Geometry: final body of the model. Coordinates: model frame, mm. A direction names the side the tool comes from. Give positions to 0.01 mm unless a question says otherwise; leave off trailing zeros. Order: outer loops, then holes, each group sorted by start corner. A loop starts at its lowest first (then second) coordinate and runs counter-clockwise, first axis right, second up. Notation, with made-up numbers: (63.25, 32.5) -> (103.25, 32.5) arc R18 cw to (103.25, 60.5) -> close; hole circle Ø10 at (48.5, 6). An arc over 180 degrees is marked (long way). Write item = value, one per line.
```python
from build123d import *

# Parameters (mm, degrees)
F0_W      = 96.012
F0_H      = 50.8
F1_DEPTH  = 56.896
F3_DEPTH  = 96.012
F5_DEPTH  = 56.896
F7_DEPTH  = 56.896
F9_DEPTH  = 31.75
F10_W     = 25.4
F10_H     = 25.4
F11_DEPTH = 19.304
F12_W     = 28.956
F12_H     = 20.32
F13_DEPTH = 13.716


with BuildPart() as f1:
    # F0 (on Front) → F1 (new body)
    with BuildSketch(Plane.XZ):
        with Locations((48.006, 25.4)):
            Rectangle(F0_W, F0_H)
    extrude(amount=F1_DEPTH)

    # F2 (on face) → F3 (cut)
    with BuildSketch(Plane.YZ.offset(96.012)):
        Polygon((-56.896, 6.604), (-12.7, 50.8), (-56.896, 50.8), align=None)
    extrude(amount=-F3_DEPTH, mode=Mode.SUBTRACT)

    # F4 (on face) → F5 (cut)
    with BuildSketch(Plane(origin=(0, 0, 0), x_dir=(-1, 0, 0), z_dir=(0, 1, 0))):
        Polygon((0, 32.004), (0, 50.8), (-57.955627, 50.8), (-25.4, 32.004), align=None)
    extrude(amount=-F5_DEPTH, mode=Mode.SUBTRACT)

    # F6 (on face) → F7 (cut)
    with BuildSketch(Plane(origin=(0, 0, 0), x_dir=(-1, 0, 0), z_dir=(0, 1, 0))):
        Polygon((-77.216, 50.8), (-96.012, 50.8), (-96.012, 32.004), align=None)
    extrude(amount=-F7_DEPTH, mode=Mode.SUBTRACT)

    # F8 (on face) → F9 (cut)
    with BuildSketch(Plane.YZ.offset(96.012)):
        with BuildLine():
            ThreePointArc((-19.304, 7.8105), (-13.69134, 10.13534), (-11.3665, 15.748))
            ThreePointArc((-11.3665, 15.748), (-24.91666, 21.36066), (-19.304, 7.8105))
        make_face()
    extrude(amount=-F9_DEPTH, mode=Mode.SUBTRACT)

    # F10 (on face) → F11 (cut)
    with BuildSketch(Plane.XZ.offset(56.896)):
        with Locations((83.312, 12.7)):
            Rectangle(F10_W, F10_H)
    extrude(amount=-F11_DEPTH, mode=Mode.SUBTRACT)

    # F12 (on face) → F13 (cut)
    with BuildSketch(Plane.XZ.offset(56.896)):
        with Locations((39.878, 10.16)):
            Rectangle(F12_W, F12_H)
    extrude(amount=-F13_DEPTH, mode=Mode.SUBTRACT)


solid = f1.part
```
1) Section query D-D (x = 10.5). Output: boundary loops of the cut face in (y, z).
Check sheet entries:
outline = (-56.9, 0) -> (0, 0) -> (0, 32) -> (-31.5, 32) -> (-56.9, 6.6) -> close
2) Line query: line 1 (X direction, y = -50, z = 11.5); line 2 (Y direction, x = 89.5, z = 15); line 3 (Y direction, x = 32, z = 15). Output: solid intervals per line, ascending. Write a range as from..to.
Check sheet entries:
line_1 = 0..25.4, 54.36..70.61
line_2 = -37.59..-27.21, -11.4..0
line_3 = -43.18..0
3) Section query B-B (x = 69). Output: boundary loops of the cut face in (y, z) (1 decimal), plus the area to 3 significant figures.
Check sheet entries:
outline = (-56.9, 0) -> (0, 0) -> (0, 50.8) -> (-12.7, 50.8) -> (-56.9, 6.6) -> close; hole circle Ø15.9 at (-19.3, 15.7)
area = 1,720 mm²
4) Reachability of faces 5 (the face through (40, -43.18, 10)), 6 (the face through (83, -37.592, 13)), 7 (the face through (13, -16, 32.004)), 8 (the face through (96.012, -14.5, 8.7)), 9 (the face through (88.834, -12.028, 39.182)) from +Z, -Z, +X, -X, +Y, -Y: full face, straight path, thin tool, end or side. Return the list, or none.
Check sheet entries:
face_5 = +Z, -Z, -Y
face_6 = -Z, +X, -Y
face_7 = +Z, -X, +Y, -Y
face_8 = +Z, -Z, +X, +Y, -Y
face_9 = +Z, +X, +Y, -Y
5) Section query A-A (y = -52.5). Output: boundary loops of the cut face in (x, z), plus the area to 3 significant figures.
Check sheet entries:
outline = (0, 0) -> (25.4, 0) -> (25.4, 11) -> (0, 11) -> close; (54.36, 0) -> (70.61, 0) -> (70.61, 11) -> (54.36, 11) -> close
area = 458 mm²
6) Section query C-C (z = 5.5). Output: boundary loops of the cut face in (x, y).
Check sheet entries:
outline = (0, -56.9) -> (25.4, -56.9) -> (25.4, -43.18) -> (54.36, -43.18) -> (54.36, -56.9) -> (70.61, -56.9) -> (70.61, -37.59) -> (96.01, -37.59) -> (96.01, 0) -> (0, 0) -> close
7) Mould query, pull axis X, two halves, no side actions, for faces 1 (the face through (25.4, -49, 8)), 2 (the face through (67, -6, 50.8)), 3 (the face through (54.356, -49, 8)), 4 (the face through (64.262, -19, 16)). Classes: +X half, -X half, draft (parallel to the pull), parting line (faces both ways), or undercut.
Check sheet entries:
face_1 = undercut
face_2 = draft
face_3 = undercut
face_4 = +X half
8) First-contact query: P1, Ø5, axis at x = 86, y = -35.5, coming from the +Z side; P2, Ø10, axis at x = 32, z = 5.5, coming from the -Y side; P3, Ø7, axis at y = -49.5, z = 5.5, coming from the +X side. Flat tips, straight axial feed; report the tip coordinate or a pass-through.
Check sheet entries:
P1 = 30.5
P2 = -43.18
P3 = 70.61
